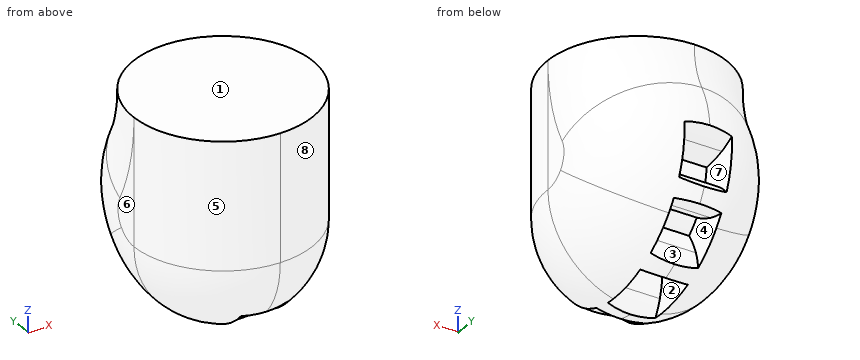
from build123d import *

# Parameters (mm, degrees)
BOSS_EXTRUDE1_DEPTH      = 18.75
BOSS_EXTRUDE1_DEPTH_BACK = 18.75
FILLET1_R                = 18.75
CUT_EXTRUDE1_DEPTH       = 5
CUT_EXTRUDE1_DEPTH_BACK  = 5


with BuildPart() as part:
    # Sketch1 → Boss-Extrude1 (new, two sides: drawn at the far end of the back side and taken through both)
    with BuildSketch(Plane(origin=(0, 0, 0), x_dir=(0, 0, -1), z_dir=(1, 0, 0)).offset(-BOSS_EXTRUDE1_DEPTH_BACK)):
        with BuildLine():
            Line((-21.199959993, 18.75), (-21.199959993, 0))
            Line((-21.199959993, 0), (24, 0))
            ThreePointArc((24, 0), (21.628103458, 10.403131298), (14.981238267, 18.75))
            Line((14.981238267, 18.75), (-21.199959993, 18.75))
        make_face()
        with BuildLine():
            ThreePointArc((-11.199959993, 21.226419768), (-16.048924785, 19.37831648), (-21.199959993, 18.75))
            Line((-21.199959993, 18.75), (14.981238267, 18.75))
            ThreePointArc((14.981238267, 18.75), (2.260017713, 23.893353049), (-11.199959993, 21.226419768))
        make_face()
        with BuildLine():
            ThreePointArc((24, 0), (18.508252147, -13.258252147), (5.25, -18.75))
            Line((5.25, -18.75), (-21.199959993, -18.75))
            Line((-21.199959993, -18.75), (-21.199959993, 0))
            Line((-21.199959993, 0), (24, 0))
        make_face()
    extrude(amount=BOSS_EXTRUDE1_DEPTH + BOSS_EXTRUDE1_DEPTH_BACK)

    # Fillet1
    fillet1_edges = [part.edges().sort_by_distance(p)[0] for p in [
        (18.75, -18.75, 7.974979997),
        (-18.75, -18.75, 7.974979997),
        (18.75, -13.258252147, -18.508252147),
        (-18.75, -13.258252147, -18.508252147),
        (18.75, 20.552360446, -12.393566076),
        (-18.75, 20.552360446, -12.393566076),
        (18.75, 19.37831648, 16.048924785),
        (-18.75, 19.37831648, 16.048924785),
    ]]
    fillet(fillet1_edges, radius=FILLET1_R - 0.0001)  # a hair under: the kernel refuses the full size

    # Sketch2 → Cut-Extrude1 (cut, two sides: drawn at the far end of the back side and taken through both)
    with BuildSketch(Plane(origin=(0, 0, 0), x_dir=(0, 0, -1), z_dir=(1, 0, 0)).offset(-CUT_EXTRUDE1_DEPTH_BACK)):
        with BuildLine():
            ThreePointArc((6.449036598, 18.931717486), (5.121740793, 16.758420159), (4.08141286, 14.434059341))
            ThreePointArc((4.08141286, 14.434059341), (2.346516976, 14.815325109), (0.578715338, 14.988832128))
            ThreePointArc((0.578715338, 14.988832128), (0.307571672, 17.520909641), (-0.283175845, 19.997995186))
            ThreePointArc((-0.283175845, 19.997995186), (-1.077578354, 22.021879435), (-2.170046216, 23.901692397))
            ThreePointArc((-2.170046216, 23.901692397), (52.177632289, 26.585831545), (18.061354181, -15.804666563))
            ThreePointArc((18.061354181, -15.804666563), (17.182690047, -13.815915161), (16.012271373, -11.983620717))
            ThreePointArc((16.012271373, -11.983620717), (14.35549975, -10.049701585), (12.466380259, -8.34202393))
            ThreePointArc((12.466380259, -8.34202393), (13.365097847, -6.809857488), (14.076393592, -5.182194847))
            ThreePointArc((14.076393592, -5.182194847), (16.568330412, -5.706776879), (19.106729783, -5.910404133))
            ThreePointArc((19.106729783, -5.910404133), (21.277041962, -5.780297079), (23.402441464, -5.322192551))
            ThreePointArc((23.402441464, -5.322192551), (23.704520174, -3.754427161), (23.901692397, -2.170046216))
            ThreePointArc((23.901692397, -2.170046216), (22.021879435, -1.077578354), (19.997995186, -0.283175845))
            ThreePointArc((19.997995186, -0.283175845), (17.520909641, 0.307571672), (14.988832128, 0.578715338))
            ThreePointArc((14.988832128, 0.578715338), (14.815325109, 2.346516975), (14.434059341, 4.08141286))
            ThreePointArc((14.434059341, 4.08141286), (16.75842016, 5.121740793), (18.931717486, 6.449036598))
            ThreePointArc((18.931717486, 6.449036598), (20.611061914, 7.829972908), (22.061279145, 9.449865739))
            ThreePointArc((22.061279145, 9.449865739), (21.384156581, 10.895771994), (20.612396506, 12.293458028))
            ThreePointArc((20.612396506, 12.293458028), (18.449459375, 12.072356759), (16.345164544, 11.525432574))
            ThreePointArc((16.345164544, 11.525432574), (13.993927564, 10.547363003), (11.786059576, 9.278405017))
            ThreePointArc((11.786059576, 9.278405017), (10.606601718, 10.606601718), (9.278405018, 11.786059576))
            ThreePointArc((9.278405018, 11.786059576), (10.547363004, 13.993927564), (11.525432575, 16.345164544))
            ThreePointArc((11.525432575, 16.345164544), (12.072356759, 18.449459375), (12.293458029, 20.612396506))
            ThreePointArc((12.293458029, 20.612396506), (10.895771994, 21.384156581), (9.449865739, 22.061279145))
            ThreePointArc((9.449865739, 22.061279145), (7.829972908, 20.611061914), (6.449036598, 18.931717486))
        make_face()
    extrude(amount=CUT_EXTRUDE1_DEPTH + CUT_EXTRUDE1_DEPTH_BACK, mode=Mode.SUBTRACT)


solid = part.part
Build history of the part. All positions in model axes, mm. Face numbers are marked on the shaded views. A direction names the side the tool comes from. Give positions to 0.01 mm unless a question says otherwise; leave off trailing zeros. Use one line per item in the form item = value.
Q1. Which spindle directions (+Z, -Z, +X, -X, +Y, -Y) get a long thin tool onto all of the face, cutting with end or side? Do the marked faces 1, 2, 3, 4 and 5. Say none if no direction does.
Conclusion:
face_1 = +Z, +X, -X, +Y, -Y
face_2 = -Z
face_3 = +Y
face_4 = none
face_5 = +Z, -Z, -X, -Y
Q2. Wall check: probe 1 along Y at (x, z) = (1.5, -17); probe 2 along X at (y, z) = (2, 10). Give the ranges that are in metal, low to high.
Conclusion:
probe_1 = -14.53 to -13.49, -5.76 to 0.39, 5.25 to 11.73
probe_2 = -18.75 to 18.75
Q3. Pin check, flat tips, straight feed: P1, Ø2.5, axis at y = 2.5, z = -21, coming from the -X side; P2, Ø11.5, axis at y = 16, z = -15.5, coming from the -X side; P3, Ø2, axis at x = -2, z = 2.5, coming from the -Y side. Stop position of each tip, or through.
Conclusion:
P1 = -11.7
P2 = -14.98
P3 = -18.72
Q4. Pull direction X, two halves, no side cores. Call the marked faces 6, 7 and 8: released by +X, released by -X, zero draft, split by the parting line, or undercut.
Conclusion:
face_6 = released by -X
face_7 = undercut
face_8 = released by +X
